Geometry: final body of the model. Coordinates: model frame, mm. Face numbers are marked on the shaded views. Round coordinates to 2 decimals unless told otherwise and drop trailing zeros. Loops run counter-clockwise (first coordinate to the right, second up) from the corner with the lowest first, then second, coordinate; pieces in that order, holes last. Notation, with made-up numbers: (87, 42.5) -> (96, 42.5) arc R7 ccw to (96, 53.5) -> close; hole circle Ø2 at (18.5, 36.5). An arc over 180 degrees is marked (long way). Answer in a Markdown table with one row per item.
```python
from build123d import *

# Parameters (mm, degrees)
F0_R        = 1.02362
F0_R_2      = 1.5875
F1_DEPTH    = 1.5875
F2_SIZE2    = 0.762
F2_SIZE     = 0.762
F3_T1_DEPTH = 5.9330773534


# Not quite as in the source:
# - a fillet or chamfer that OpenCascade refuses, or shapes differently, is made with other operations: its cross-section is extruded or revolved along the edge and cut away or added


with BuildPart() as f1:
    # F0 (on Front) → F1 (new body, symmetric)
    with BuildSketch(Plane.XZ):
        with BuildLine():
            Line((-6.9308998718, -2.1542398912), (-5.8992384492, -1.5586098912))
            Line((-5.8992384492, -1.5586098912), (-3.5910470257, -5.5565147104))
            ThreePointArc((-3.5910470257, -5.5565147104), (8.1172314393, 9.2773759439), (-6.9308998718, -2.1542398912))
        make_face()
        with Locations((7.9313591488, -0.3737701657)):
            Circle(F0_R, mode=Mode.SUBTRACT)
        with Locations((1.3199729119, 2.6048275917)):
            Circle(F0_R_2, mode=Mode.SUBTRACT)
    extrude(amount=F1_DEPTH, both=True)

    # F2
    f2_edges = [f1.edges().sort_by_distance(p)[0] for p in [
        (6.907739, -1.5875, -0.37377),
    ]]
    chamfer(f2_edges, length=F2_SIZE, length2=F2_SIZE2)

    # F3: chamfer of 0.508 on 1 edges, made by hand

    # F3_s2 → F3_t1 (cut)
    with BuildSketch(Plane.XZ.offset(-2.9665386767)):
        with BuildLine():
            Line((-6.4783627065, -1.892967437), (-7.1860154174, -1.6816380318))
            ThreePointArc((-7.1860154174, -1.6816380318), (-7.0651975677, -1.9134177566), (-6.9308998718, -2.1542398912))
            Line((-6.9308998718, -2.1542398912), (-6.4783627065, -1.892967437))
        make_face()
    extrude(amount=F3_T1_DEPTH, mode=Mode.SUBTRACT)


solid = f1.part
```
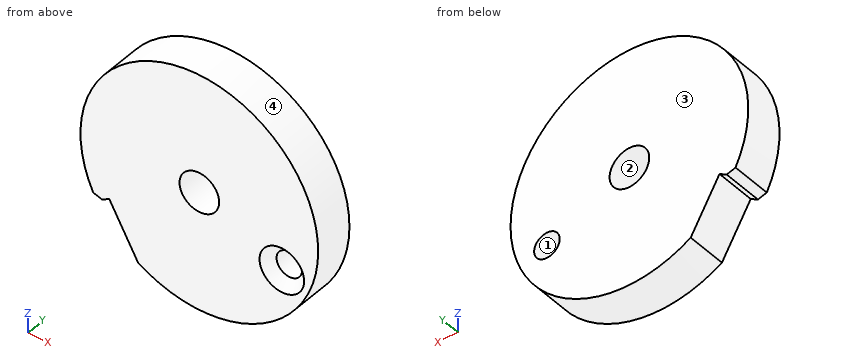
Item 1: Section query D-D, the plane x = 5.5. Output: boundary loops of the cut face in (y, z).
Ans:
| item | result |
|---|---|
| outline | (-1.59, -5.95) -> (1.59, -5.95) -> (1.59, 11.16) -> (-1.59, 11.16) -> close |
Item 2: Ray query, L1, parallel to Z at x = 2.25, y = -1.4; L2, parallel to Z at x = 8, y = -1; L3, parallel to X at y = 1.15, z = 3.25. Return the intervals inside material, ascending.
Ans:
| item | result |
|---|---|
| L1 | -6.87 to 1.32, 3.89 to 12.08 |
| L2 | -4.19 to -1.57, 0.82 to 9.39 |
| L3 | -8.18 to -0.13, 2.77 to 10.82 |
Item 3: Section query A-A, the plane x = 0.25. Output: boundary loops of the cut face in (y, z), and give its area (3 significant figures).
Ans:
| item | result |
|---|---|
| outline | (-1.59, -6.86) -> (1.59, -6.86) -> (1.59, 1.43) -> (-1.59, 1.43) -> close; (-1.59, 3.78) -> (1.59, 3.78) -> (1.59, 12.07) -> (-1.59, 12.07) -> close |
| area | 52.7 mm2 |
Item 4: Section query C-C, the plane y = 1.1. State how many separate pieces and enclosed holes the cut face has, and give its area (3 significant figures).
Ans:
| item | result |
|---|---|
| separate pieces | 1 |
| enclosed holes | 2 |
| area | 270 mm2 |
Item 5: Section query B-B, the plane z = 2. Output: boundary loops of the cut face in (x, y).
Ans:
| item | result |
|---|---|
| outline | (-8.19, -1.59) -> (-0.15, -1.59) -> (-0.15, 1.59) -> (-8.19, 1.59) -> close; (2.79, -1.59) -> (10.83, -1.59) -> (10.83, 1.59) -> (2.79, 1.59) -> close |
Item 6: Mould query, pull axis X, two halves, no side actions, for the marked faces 1, 2, 3 and 4. Classes: released by +X, released by -X, zero draft, split by the parting line, or undercut.
Ans:
| item | result |
|---|---|
| face 1 | undercut |
| face 2 | undercut |
| face 3 | zero draft |
| face 4 | split by the parting line |
Item 7: First-contact query: P1, Ø2.5, axis at x = 7.93, z = -0.37, coming from the -Y side; P2, Ø2.5, axis at x = 1.32, z = 2.6, coming from the -Y side; P3, Ø5, axis at x = 8, z = 9.5, coming from the -Y side; P4, Ø1, axis at x = 8.5, y = 0.5, coming from the +Z side. Flat tips, straight axial feed; report the tip coordinate or a pass-through.
Ans:
| item | result |
|---|---|
| P1 | y = -1.06 |
| P2 | through |
| P3 | y = -1.59 |
| P4 | z = 9.39 |
